For this review, take the finished solid that the model builds, in its own axes (mm). A direction names the side the tool comes from. Round coordinates to 2 decimals unless told otherwise and drop trailing zeros. Write each loop counter-clockwise with the first axis right and the second up, starting at its lowest first coordinate (ties: lowest second). Pieces come first, ordered by that corner, then holes. Notation, with made-up numbers: (-26.75, 76) - (19.25, 76) arc R35 cw to (19.25, 108) - close; hole circle Ø2 at (85, -34). An arc over 180 degrees is marked (long way). Answer in a Markdown table with one row per item. Add a question column.
Autodesk Inventor part; units mm, degrees
ref_plane "YZ Plane" through (0, 0, 0) normal (1, 0, 0) x (0, 1, 0)
ref_plane "XZ Plane" through (0, 0, 0) normal (0, 1, 0) x (-1, 0, 0)
sketch "Skizze1" plane through (0, 0, 0) normal (0, 0, 1) x (1, 0, 0)
  line L0 (0, 0) -> (0, 5)
  line L1 (0, 5) -> (0.8, 5)
  line L2 (0.8, 5) -> (0.8, 4.8)
  line L3 (0.8, 4.8) -> (1.9, 4.8)
  line L4 (1.9, 4.8) -> (1.9, 5)
  line L5 (1.9, 5) -> (24.9, 5)
  line L6 (24.9, 5) -> (24.9, 7.25)
  line L7 (24.9, 7.25) -> (30.9, 7.25)
  line L8 (30.9, 7.25) -> (30.9, 5)
  line L9 (30.9, 5) -> (53.9, 5)
  line L10 (53.9, 5) -> (53.9, 4)
  line L11 (53.9, 4) -> (63.1, 4)
  line L12 (63.1, 4) -> (63.1, 0)
  line L13 (63.1, 0) -> (0, 0)
  line L14 (15.9, 5) -> (15.9, 0) construction
  line L15 (39.9, 5) -> (39.9, 0) construction
  line L16 (9.9, 5) -> (9.9, 0) construction
  line L17 (45.9, 5) -> (45.9, 0) construction
  line L18 (53.9, 5) -> (53.9, 0) construction
  dimension "d0" = 10
  dimension "d2" = 14.5
  dimension "d3" = 1.1
  dimension "d4" = 9.6
  dimension "d5" = 0.8
  dimension "d7" = 9
  dimension "d8" = 9
  dimension "d9" = 6
  dimension "d10" = 14
  dimension "d11" = 14
  dimension "ParrallelMecha_DrivenLink_OuterWidth" = 52
  dimension "d22" = 6
  dimension "d23" = 6
  dimension "Querstrebe_Length" = 36
  dimension "d25" = 9.2
  dimension "d26" = 8
revolve "Umdrehung1" add sketch "Skizze1" angle 360 about axis through (63.1, 0, 0) along (-1, 0, 0)
chamfer "Fase1" distance 0.2 angle 45 4 edges at (24.9, -7.25, 0) (30.9, -7.25, 0) (63.1, -4, 0) (0, -5, 0)
ref_plane "Wellennut_Spiegelebene" through (27.9, 0, 0) normal (-1, 0, 0) x (0, 0, 1)
ref_plane "Arbeitsebene2" through (13.4, 0, 5) normal (0, 0, 1) x (1, 0, 0)
sketch "Skizze3" plane through (13.4, 0, 5) normal (0, 0, 1) x (1, 0, 0)
  line L0 (2.5, 5) -> (2.5, 0) construction
  line L1 (-26.02, 0) -> (62.32, 0) construction
  line L2 (0, 0) -> (-9, 0) construction
  line L3 (0, 1.5) -> (-9, 1.5)
  line L4 (-9, -1.5) -> (0, -1.5)
  arc A0 (0, -1.5) -> (0, 1.5) centre (0, 0) ccw
  arc A1 (-9, 1.5) -> (-9, -1.5) centre (-9, 0) ccw
  line L5 (-11.5, 0) -> (2.5, 0) construction
  line L6 (-11.5, -5) -> (-11.5, 5) construction
  point P0 (-13.4, 0)
  point P1 (-4.5, 0)
  point P2 (-4.5, 0)
  dimension "d17" = 3
  dimension "d18" = 12
extrude "Wellennut" cut sketch "Skizze3" against normal blind 1.8
mirror "Spiegeln1" about plane through (27.9, 0, 0) normal (-1, 0, 0) of "Wellennut"
sketch "Skizze4" plane through (53.9, 0, 0) normal (1, 0, 0) x (0, 0, -1)
  circle A0 centre (0, 0) radius 4
  line L0 (-3, -2.6458) -> (-3, 2.6458)
  point P0 (0, 0)
  dimension "d27" = 3
extrude "Extrusion2" cut sketch "Skizze4" along normal through all contours L0 A0 picked at (-3.1815, -0.6179)
chamfer "Fase2" distance 0.2 angle 45 1 edges at (63.1, 0, 3)
sketch "Skizze5" plane through (63.1, 0, 0) normal (1, 0, 0) x (0, 0, -1)
  arc A0 (-3, -2.6458) -> (-3, 2.6458) centre (0, 0) ccw construction
  circle A1 centre (0, 0) radius 5 construction
  point P0 (0, 0)
hole "Bohrung1" at (63.1, 0, 0) direction (-1, 0, 0) diameter 2.459 depth 8 tip angle 118
chamfer "Fase3" distance 0.5 angle 45 1 edges at (63.1, 0, 1.2295)
equation "\"d10\" = ParallelLink_Lever_Thickness + ParallelMecha_Bearing_Step_Thickness"
equation "\"d11\" = d10"
equation "\"d22\" = ParallelMecha_Bearing_Step_Thickness"
equation "\"d23\" = d22"
equation "\"d26\" = CapstonV2_ShaftDia"
properties part number "ParallelSystem_ProximalPart_Shaft_Driven_Rillenkugellager" material "Edelstahl"
Q1. Tool access review of faces 1 (the face through (58, 0, 3)), 2 (the face through (52.9, 0, 4.1)), 3 (the face through (42.56, -1.08, -4.88)): name each direction out of +Z, -Z, +X, -X, +Y, -Y from which nothing blocks a thin tool from reaching the whole face with its end or side.
Q2. Add section A-A on x = 58.5. State the section outline as (y, z) points, then the cut area to 3 significant figures.
Q3. Add section B-B on x = 7.5. State the section outline as (y, z) points, then the cut area to 3 significant figures.
Q4. To check wall thickness, follow probe 1 along Y at (x, z) = (57.5, 0); probe 2 along Z at (x, y) = (58.5, 0); probe 3 along X at (y, z) = (0, 4.75). State the ranges of each line that lie inside material, in increasing order.
Q5. Draft analysis for pull direction Z (two halves, no side actions). For faces 4 (the face through (1.36, 2.58, 4.05)), 5 (the face through (58.798, 0.748, 0.976)), 6 (the face through (53.9, 0, 3.3)), state which applies: released by +Z, released by -Z, zero draft, split by the parting line, or undercut.
Q6. Add section C-C on z = 4. Count the separate pieces of the cut face and the enclosed holes in it, then the cut area to 3 significant figures.
Q7. Insertion check: pin 1 Ø2.5 at (x, y) = (57, 0) entering from +Z; pin 2 Ø1.3 at (x, z) = (44.5, 4) entering from -Y; pin 3 Ø1.7 at (x, z) = (45.5, 4) entering from +Y. Each pin has a flat end and moves straight along its axis. Give the tip position at first contact, or say it passes through.
Answer sheet:
| question | item | result |
|---|---|---|
| 1 | face 1 | +Z, +X, +Y, -Y |
| 1 | face 2 | +Z |
| 1 | face 3 | +X |
| 2 | outline | (-2.65, 3) arc R4 ccw (long way) to (2.65, 3) - close; hole circle Ø2.46 at (0, 0) |
| 2 | area | 41.9 mm² |
| 3 | outline | (-1.5, 3.2) - (-1.5, 4.77) arc R5 ccw (long way) to (1.5, 4.77) - (1.5, 3.2) - close |
| 3 | area | 73.4 mm² |
| 4 | probe 1 | y = -4 to -1.23, 1.23 to 4 |
| 4 | probe 2 | z = -4 to -1.23, 1.23 to 3 |
| 4 | probe 3 | x = 0 to 2.9, 14.9 to 40.9, 52.9 to 53.9 |
| 5 | face 4 | split by the parting line |
| 5 | face 5 | undercut |
| 5 | face 6 | zero draft |
| 6 | separate pieces | 1 |
| 6 | enclosed holes | 2 |
| 6 | area | 291 mm² |
| 7 | pin 1 | stops at z = 3 |
| 7 | pin 2 | stops at y = -3.71 |
| 7 | pin 3 | stops at y = 3.88 |
